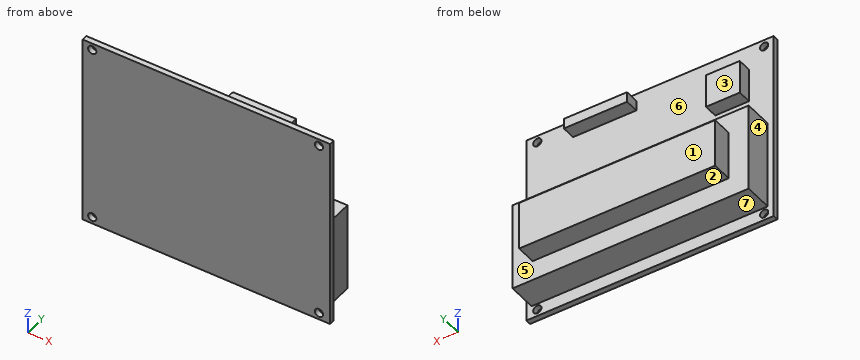
```python
from build123d import *

# Parameters (mm, degrees)
SKETCH1_W           = 90
SKETCH1_H           = 70
BOSS_EXTRUDE1_DEPTH = 2
SKETCH2_R           = 1.5
CUT_EXTRUDE1_DEPTH  = 3
SKETCH3_W           = 23
SKETCH3_H           = 3.733741838
SKETCH3_W_2         = 12.3
SKETCH3_H_2         = 12.3
BOSS_EXTRUDE2_DEPTH = 5
SKETCH4_W           = 71.3
SKETCH4_H           = 17.735180651
BOSS_EXTRUDE3_DEPTH = 17.6
SKETCH5_W           = 85.9
SKETCH5_H           = 32.335180651
BOSS_EXTRUDE4_DEPTH = 10.3


with BuildPart() as part:
    # Sketch1 → Boss-Extrude1 (new body)
    with BuildSketch(Plane(origin=(0, 0, 0), x_dir=(1, 0, 0), z_dir=(0, 1, 0))):
        Rectangle(SKETCH1_W, SKETCH1_H)
    extrude(amount=BOSS_EXTRUDE1_DEPTH)

    # Sketch2 → Cut-Extrude1 (cut, through all)
    with BuildSketch(Plane(origin=(0, 2, 0), x_dir=(1, 0, 0), z_dir=(0, 1, 0))):
        with Locations((-41.5, 32.5)):
            Circle(SKETCH2_R)
        with Locations((-41.5, -32.5)):
            Circle(SKETCH2_R)
        with Locations((41, -32.5)):
            Circle(SKETCH2_R)
        with Locations((41, 32.5)):
            Circle(SKETCH2_R)
    extrude(amount=-CUT_EXTRUDE1_DEPTH, mode=Mode.SUBTRACT)

    # Sketch3 → Boss-Extrude2 (add)
    with BuildSketch(Plane(origin=(0, 2, 0), x_dir=(1, 0, 0), z_dir=(0, 1, 0))):
        with Locations((16.5, -30.528214904)):
            Rectangle(SKETCH3_W, SKETCH3_H)
        with Locations((-29.85, -19.85)):
            Rectangle(SKETCH3_W_2, SKETCH3_H_2)
    extrude(amount=BOSS_EXTRUDE2_DEPTH)

    # Sketch4 → Boss-Extrude3 (add)
    with BuildSketch(Plane(origin=(0, 2, 0), x_dir=(1, 0, 0), z_dir=(0, 1, 0))):
        with Locations((0.15, 14.132409674)):
            Rectangle(SKETCH4_W, SKETCH4_H)
    extrude(amount=BOSS_EXTRUDE3_DEPTH)

    # Sketch5 → Boss-Extrude4 (add)
    with BuildSketch(Plane(origin=(0, 2, 0), x_dir=(1, 0, 0), z_dir=(0, 1, 0))):
        with Locations((0.15, 14.132409674)):
            Rectangle(SKETCH5_W, SKETCH5_H)
    extrude(amount=BOSS_EXTRUDE4_DEPTH)


solid = part.part
```
Build history of the part. All positions in model axes, mm. Face numbers are marked on the shaded views. A direction names the side the tool comes from. Give positions to 0.01 mm unless a question says otherwise; leave off trailing zeros. Loops run counter-clockwise (first coordinate to the right, second up) from the corner with the lowest first, then second, coordinate; pieces in that order, holes last. Notation, with made-up numbers: (31.5, 2) -> (43.5, 2) arc R14 ccw to (43.5, 15) -> close; hole circle Ø10 at (75.5, -11). An arc over 180 degrees is marked (long way). One line per question, with ' | ' between items.
Q1. Cut at B-B, the plane x = 41. Write the cut outline in (y, z).
Filled sheet:
outline: (0, -35) -> (2, -35) -> (2, -34) -> (0, -34) -> close; (0, -31) -> (2, -31) -> (2, -30.3) -> (12.3, -30.3) -> (12.3, 2.04) -> (2, 2.04) -> (2, 31) -> (0, 31) -> close; (0, 34) -> (2, 34) -> (2, 35) -> (0, 35) -> close
Q2. Pull direction Z, two halves, no side cores. Call the marked faces 5, 6 and 7: pulls with the +Z half, pulls with the -Z half, needs draft (parallel to the pull), parting line crosses it, or undercut.
Filled sheet:
face 5: needs draft | face 6: undercut | face 7: pulls with the -Z half
Q3. Drop flat-ended pins along their axis: pin 1 (8 mm diameter, centred on y = 9, z = -8, fed in from -X); pin 2 (3.5 mm diameter, centred on y = 16.5, z = -16, fed in from -X); pin 3 (6 mm diameter, centred on y = 14.5, z = -16.5, fed in from +X). Give the stop position or say it passes through.
Filled sheet:
pin 1: stops at x = -42.8 | pin 2: stops at x = -35.5 | pin 3: stops at x = 43.1
Q4. Drill centre lines: line 1 along Z through (x, y) = (41, 1.55); line 2 along X through (y, z) = (0.45, 32.5); line 3 along X through (y, z) = (10, -29.5). Where is each one in solid material? Low to high. Write a range as [from, to].
Filled sheet:
line 1: z = [-35, -34], [-31, 31], [34, 35] | line 2: x = [-45, -43], [-40, 39.5], [42.5, 45] | line 3: x = [-42.8, 43.1]
Q5. Tool access for the marked faces 1, 2, 3 and 4: list every direction of +Z, -Z, +X, -X, +Y, -Y with a clear straight run to the whole face (end or side of a thin tool).
Filled sheet:
face 1: +Z, -Z, +X, -X, +Y | face 2: -Z, +X, -X, +Y | face 3: +Z, +X, -X, +Y | face 4: +Z, -Z, -X, +Y
Q6. Cut at A-A, the plane z = -32.5. Write the cut outline in (x, y).
Filled sheet:
outline: (-45, 0) -> (-43, 0) -> (-43, 2) -> (-45, 2) -> close; (-40, 0) -> (39.5, 0) -> (39.5, 2) -> (-40, 2) -> close; (42.5, 0) -> (45, 0) -> (45, 2) -> (42.5, 2) -> close
Q7. Cut at D-D, the plane x = -27. Write the cut outline in (y, z).
Filled sheet:
outline: (0, -35) -> (2, -35) -> (2, -30.3) -> (12.3, -30.3) -> (12.3, -23) -> (19.6, -23) -> (19.6, -5.26) -> (12.3, -5.26) -> (12.3, 2.04) -> (2, 2.04) -> (2, 13.7) -> (7, 13.7) -> (7, 26) -> (2, 26) -> (2, 35) -> (0, 35) -> close
Q8. Cut at C-C, the plane y = 4.5. Write the cut outline in (x, z).
Filled sheet:
outline: (-42.8, -30.3) -> (43.1, -30.3) -> (43.1, 2.04) -> (-42.8, 2.04) -> close; (-36, 13.7) -> (-23.7, 13.7) -> (-23.7, 26) -> (-36, 26) -> close; (5, 28.66) -> (28, 28.66) -> (28, 32.4) -> (5, 32.4) -> close
